The model under review builds one solid part; all positions refer to its coordinate system, in mm. Face numbers are marked on the shaded views. A direction names the side the tool comes from. Coordinates: 2 decimals unless noted, no trailing zeros. Write each loop counter-clockwise with the first axis right and the second up, starting at its lowest first coordinate (ties: lowest second). Pieces come first, ordered by that corner, then holes. Notation, with made-up numbers: (3, -2.75) - (32, -2.75) arc R17 cw to (32, 2.25) - close; hole circle Ø4 at (14, 4.25). An arc over 180 degrees is marked (long way). Return JSON: item names as keys, results as strings. Group by question number.
(1) To check wall thickness, follow L1, parallel to Y at x = 51.75, z = -25; L2, parallel to Y at x = 12, z = 30; L3, parallel to Y at x = -16.5, z = -1. State the ranges of each line that lie inside material, in increasing order. Write a range as from..to.
(2) We need section B-B on x = 46. State the section outline as (y, z) points, then the cut area to 3 significant figures.
(3) We need section C-C on z = -25. State the section outline as (x, y) points.
(4) Draft analysis for pull direction X (two halves, no side actions). For the marked faces 1, 2 and 3, state which applies: released by +X, released by -X, zero draft, split by the parting line, or undercut.
(5) We need section A-A on y = 6. State the section outline as (x, z) points, then the cut area to 3 significant figures.
(6) We need section D-D on y = -1. State the section outline as (x, z) points, then the cut area to 3 significant figures.
(7) Tool access review of the marked faces 4 and 5: name each direction out of +Z, -Z, +X, -X, +Y, -Y from which nothing blocks a thin tool from reaching the whole face with its end or side.
(8) For pin 1 Ø8 at (x, z) = (23.5, -26.5) entering from +Y; pin 2 Ø5 at (y, z) = (22, -25) entering from +X; pin 3 Ø9 at (y, z) = (11, -17.5) entering from -X; pin 4 Ø2.5 at (y, z) = (22, 25) entering from -X, all flat-tipped, find the tip position at first contact; note any pin that passes through.
```python
from build123d import *

# Parameters (mm, degrees)
EXTRUDE_1_DEPTH     = 10.4
SKETCH_2_W          = 10.2
SKETCH_2_H          = 70
EXTRUDE_2_DEPTH     = 30
SKETCH_3_R          = 2.1
CUT_EXTRUDE_3_DEPTH = 102.118742081
SKETCH_4_R          = 20
CUT_EXTRUDE_4_DEPTH = 2


with BuildPart() as part:
    # Sketch 1 → Extrude 1 (new body)
    with BuildSketch(Plane(origin=(0, 0, 0), x_dir=(1, 0, 0), z_dir=(0, 1, 0))):
        with BuildLine():
            Line((0, 35), (55, 35))
            Line((55, 35), (55, -35))
            Line((55, -35), (0, -35))
            ThreePointArc((0, -35), (-35, 0), (0, 35))
        make_face()
    extrude(amount=-EXTRUDE_1_DEPTH)

    # Sketch 2 → Extrude 2 (add)
    with BuildSketch(Plane(origin=(0, 0, 0), x_dir=(-1, 0, 0), z_dir=(0, -1, 0))):
        with Locations((-49.9, 0)):
            Rectangle(SKETCH_2_W, SKETCH_2_H)
    extrude(amount=-EXTRUDE_2_DEPTH)

    # Sketch 3 → Cut-Extrude 3 (cut, through all)
    with BuildSketch(Plane(origin=(55, 0, 0), x_dir=(0, 0, -1), z_dir=(1, 0, 0))):
        with Locations((25, 22)):
            Circle(SKETCH_3_R)
        with Locations((25, 6)):
            Circle(SKETCH_3_R)
        with Locations((-25, 6)):
            Circle(SKETCH_3_R)
        with Locations((-25, 22)):
            Circle(SKETCH_3_R)
    extrude(amount=-CUT_EXTRUDE_3_DEPTH, mode=Mode.SUBTRACT)

    # Sketch 4 → Cut-Extrude 4 (cut)
    with BuildSketch(Plane(origin=(0, 0, 0), x_dir=(1, 0, 0), z_dir=(0, 1, 0))):
        with Locations(Location((0, 0, 0), (0, 0, 270))):
            Circle(SKETCH_4_R)
    extrude(amount=-CUT_EXTRUDE_4_DEPTH, mode=Mode.SUBTRACT)


solid = part.part
```
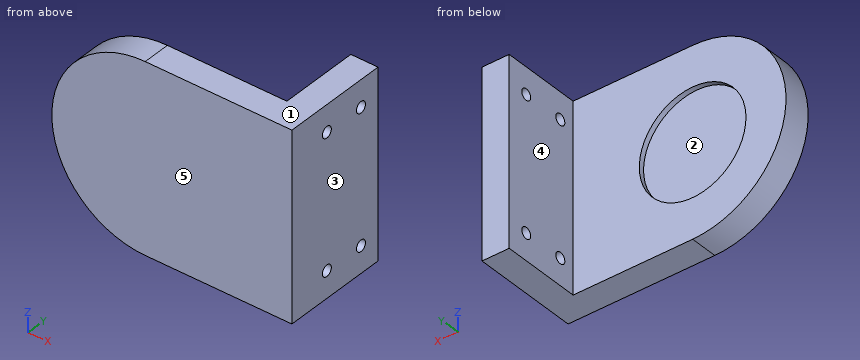
Ans:
{
 "1": {"L1": "-10.4..3.9, 8.1..19.9, 24.1..30", "L2": "-10.4..0", "L3": "-10.4..-2"},
 "2": {"outline": "(-10.4, -35) - (30, -35) - (30, 35) - (-10.4, 35) - close; hole circle Ø4.2 at (6, -25); hole circle Ø4.2 at (6, 25); hole circle Ø4.2 at (22, -25); hole circle Ø4.2 at (22, 25)", "area": "2,770 mm²"},
 "3": {"outline": "(-24.49, -10.4) - (55, -10.4) - (55, 3.9) - (44.8, 3.9) - (44.8, 0) - (-24.49, 0) - close; (44.8, 8.1) - (55, 8.1) - (55, 19.9) - (44.8, 19.9) - close; (44.8, 24.1) - (55, 24.1) - (55, 30) - (44.8, 30) - close"},
 "4": {"face 1": "zero draft", "face 2": "undercut", "face 3": "released by +X"},
 "5": {"outline": "(44.8, -35) - (55, -35) - (55, -27.1) - (44.8, -27.1) - close; (44.8, -22.9) - (55, -22.9) - (55, 22.9) - (44.8, 22.9) - close; (44.8, 27.1) - (55, 27.1) - (55, 35) - (44.8, 35) - close", "area": "628 mm²"},
 "6": {"outline": "(0, -35) - (55, -35) - (55, 35) - (0, 35) arc R35 ccw to start; hole circle Ø40 at (0, 0)", "area": "4,520 mm²"},
 "7": {"face 4": "+Z, -Z, -X, +Y", "face 5": "+Z, -Z, +X, -X, -Y"},
 "8": {"pin 1": "y = 0", "pin 2": "x = 55", "pin 3": "x = 44.8", "pin 4": "through"}
}
